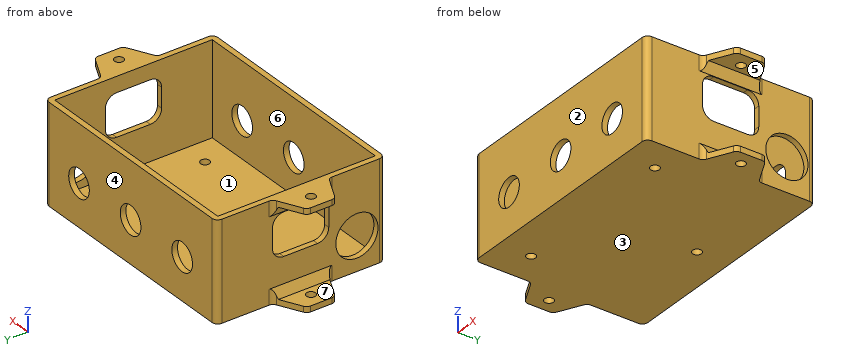
Autodesk Inventor part; units mm, degrees
ref_plane "Plano de trabajo1" through (41.5, -14.7294, 17.5) normal (0, 0, 1) x (1, 0, 0)
ref_plane "YZ Plane" through (0, 0, 0) normal (1, 0, 0) x (0, 1, 0)
ref_plane "XZ Plane" through (0, 0, 0) normal (0, 1, 0) x (-1, 0, 0)
sketch "Base" plane through (0, 0, 0) normal (0, 0, 1) x (1, 0, 0)
  line L0 (-41.5, -30) -> (41.5, -30)
  line L1 (41.5, -30) -> (41.5, -11.2361)
  line L2 (41.5, 30) -> (-41.5, 30)
  line L3 (-41.5, -30) -> (41.5, 30) construction
  line L4 (41.5, -30) -> (-41.5, 30) construction
  line L5 (-39.5, -28) -> (39.5, -28)
  line L6 (39.5, -28) -> (39.5, 28)
  line L7 (39.5, 28) -> (-39.5, 28)
  line L8 (-39.5, 28) -> (-39.5, -28)
  circle A0 centre (-30, -18.5) radius 1.35
  circle A1 centre (30, -18.5) radius 1.35
  circle A2 centre (0, 18.5) radius 1.35
  line L9 (51.5, 3.7639) -> (51.5, -3.7639)
  line L10 (41.5, 5) -> (51.5, -5) construction
  line L11 (51.5, 5) -> (41.5, -5) construction
  line L12 (42.6056, -9.4472) -> (50.3944, -5.5528)
  line L13 (50.3944, 5.5528) -> (42.6056, 9.4472)
  arc A3 (51.5, 3.7639) -> (50.3944, 5.5528) centre (49.5, 3.7639) ccw
  arc A4 (50.3944, -5.5528) -> (51.5, -3.7639) centre (49.5, -3.7639) ccw
  arc A5 (42.6056, -9.4472) -> (41.5, -11.2361) centre (43.5, -11.2361) ccw
  line L14 (41.5, 11.2361) -> (41.5, 30)
  arc A6 (41.5, 11.2361) -> (42.6056, 9.4472) centre (43.5, 11.2361) ccw
  line L15 (-41.5, -30) -> (-41.5, -11.2361)
  line L16 (-39.5, -28) -> (-39.5, 28)
  line L17 (-51.5, 3.7639) -> (-51.5, -3.7639)
  line L18 (-41.5, 5) -> (-51.5, -5) construction
  line L19 (-51.5, 5) -> (-41.5, -5) construction
  line L20 (-42.6056, -9.4472) -> (-50.3944, -5.5528)
  line L21 (-50.3944, 5.5528) -> (-42.6056, 9.4472)
  arc A7 (-50.3944, 5.5528) -> (-51.5, 3.7639) centre (-49.5, 3.7639) ccw
  arc A8 (-51.5, -3.7639) -> (-50.3944, -5.5528) centre (-49.5, -3.7639) ccw
  arc A9 (-41.5, -11.2361) -> (-42.6056, -9.4472) centre (-43.5, -11.2361) ccw
  line L22 (-41.5, 11.2361) -> (-41.5, 30)
  arc A10 (-42.6056, 9.4472) -> (-41.5, 11.2361) centre (-43.5, 11.2361) ccw
  line L23 (41.5, 11.2361) -> (41.5, -11.2361)
  line L24 (-41.5, -11.2361) -> (-41.5, 11.2361)
  circle A11 centre (-46.5, 0) radius 1.35
  circle A12 centre (46.5, 0) radius 1.35
  circle A13 centre (0, 18.5) radius 1.6
  circle A14 centre (30, -18.5) radius 1.6
  circle A15 centre (-30, -18.5) radius 1.6
  circle A16 centre (-46.5, 0) radius 1.6
  circle A17 centre (46.5, 0) radius 1.6
  point P0 (0, 0)
  point P1 (41.5, 10)
  point P2 (-41.5, 10)
  point P3 (-41.5, -10)
  point P4 (-41.5, 10)
  dimension "d0" = 83
  dimension "d1" = 60
  dimension "d5" = 2.7
  dimension "d6" = 9.5
  dimension "d8" = 2.7
  dimension "d9" = 5
  dimension "d10" = 10
  dimension "d11" = 10
  dimension "d14" = 2
  dimension "d15" = 2
  dimension "d16" = 2.7
  dimension "d17" = 2.7
  dimension "d63" = 3.2
  dimension "d64" = 3.2
  dimension "d65" = 3.2
  dimension "d66" = 3.2
  dimension "d67" = 3.2
extrude "Extrusión1" add sketch "Base" along normal blind 2 contours L8 L7 L6 L5 | A13 | A14 | A15
extrude "Extrusión2" add sketch "Base" along normal blind 2 contours A9 L20 A8 L17 A7 L21 A10 L24 | L23 A6 L13 A3 L9 A4 L12 A5 | A16 | A17
extrude "Extrusión3" cut sketch "Base" along normal blind 35 contours L15 L24 L22 L2 L14 L23 L1 L0
extrude "Extrusión4" add sketch "Base" along normal blind 35 contours L15 L24 L22 L2 L14 L23 L1 L0
sketch "Boceto2" plane through (-41.5, 30, 0) normal (0, 1, 0) x (1, 0, 0)
  line L0 (41.5, 0) -> (41.5, -35)
  line L1 (2, -35) -> (81, -35)
  line L2 (83, 0) -> (0, 0)
  circle A0 centre (16.5, -14.9) radius 5
  circle A1 centre (66.5, -14.9) radius 5
  circle A2 centre (41.5, -14.9) radius 5
  dimension "d26" = 14.9
  dimension "d27" = 25
  dimension "d28" = 10
  dimension "d29" = 10
extrude "Extrusión5" cut sketch "Boceto2" against normal blind 70
sketch "Boceto3" plane through (41.5, 11.2361, 0) normal (1, 0, 0) x (0, 0, -1)
  line L0 (-2, -39.2361) -> (-35, -39.2361)
  line L1 (-2, -15) -> (-2, -7.4721)
  line L2 (0, 0) -> (0, 18.7639)
  line L3 (-18.5, -21.2361) -> (-25.5, -21.2361)
  line L4 (-29.5, -17.2361) -> (-29.5, -5.2361)
  line L5 (-25.5, -1.2361) -> (-18.5, -1.2361)
  line L6 (-14.5, -5.2361) -> (-14.5, -17.2361)
  line L7 (-14.5, -21.2361) -> (-29.5, -1.2361) construction
  line L8 (-29.5, -21.2361) -> (-14.5, -1.2361) construction
  arc A0 (-29.5, -17.2361) -> (-25.5, -21.2361) centre (-25.5, -17.2361) ccw
  arc A1 (-18.5, -21.2361) -> (-14.5, -17.2361) centre (-18.5, -17.2361) ccw
  arc A2 (-14.5, -5.2361) -> (-18.5, -1.2361) centre (-18.5, -5.2361) ccw
  arc A3 (-25.5, -1.2361) -> (-29.5, -5.2361) centre (-25.5, -5.2361) ccw
  circle A4 centre (-12, 8.7639) radius 7.5
  point P0 (0, -11.2361)
  point P1 (-22, -11.2361)
  dimension "d32" = 28
  dimension "d33" = 48
  dimension "d34" = 20
  dimension "d35" = 12
  dimension "d36" = 15
  dimension "d37" = 20
  dimension "d38" = 4
  dimension "d39" = 15
extrude "Extrusión6" cut sketch "Boceto3" against normal blind 10
sketch3d "Boceto 3D1"
pattern_circular "Patrón circular1" count 2 over 360 about axis through (0, 0, 99.8627) along (0, 0, -1) of "Extrusión6"
sketch "Boceto4" plane through (41.5, 11.2361, 0) normal (1, 0, 0) x (0, 0, -1)
  line L0 (-35, -41.2361) -> (-35, 18.7639)
  point P0 (0, -11.2361)
  point P1 (-17.5, -25.9654)
  dimension "d45" = 17.5
ref_plane "Plano de trabajo1" through (41.5, -14.7294, 17.5) normal (0, 0, 1) x (1, 0, 0)
mirror "Simetría1" about plane through (41.5, -14.7294, 17.5) normal (0, 0, 1) of "Extrusión2"
chamfer "Chaflán1" distance 1.7 angle 63 1 edges at (41.5, 0, 33) measured on face at (43.0002, 0, 33)
mirror "Simetría2" about plane through (41.5, -14.7294, 17.5) normal (0, 0, 1) of "Extrusión2", "Simetría1", "Chaflán1"
chamfer "Chaflán2" distance 1.7 angle 63 1 edges at (-41.5, 0, 33) measured on face at (-43.0002, 0, 33)
chamfer "Chaflán3" distance 1.7 angle 63 1 edges at (-41.5, 0, 2) measured on face at (-43.0002, 0, 2)
fillet "Empalme1" radius 2 4 edges at (-41.5, 30, 17.5) (41.5, 30, 17.5) (41.5, -30, 17.5) (-41.5, -30, 17.5)
hole "Agujero2" at (0, 18.5, 0) at (-30, -18.5, 0) at (-46.5, 0, 0) at (30, -18.5, 0) at (46.5, 0, 0) direction (0, 0, 1) diameter 3.2 depth 23.25 tip angle 118
extrude "Extrusión8" cut sketch "Base" along normal blind 94.8 contours A16 | A17
properties part number "Contenedor del Arduino v1.1"
Input: part model. Units: mm. Frame: model coordinates. Face numbers are marked on the shaded views. A direction names the side the tool comes from. Give positions to 0.01 mm unless a question says otherwise; leave off trailing zeros. Loops run counter-clockwise (first coordinate to the right, second up) from the corner with the lowest first, then second, coordinate; pieces in that order, holes last. Notation, with made-up numbers: (51, 68) - (65, 68) arc R24 cw to (65, 104) - close; hole circle Ø6 at (26, -9). An arc over 180 degrees is marked (long way). Use CSV: the item, a comma, the result in double quotes. Start each with the question number.
Item 1: Mould query, pull axis Y, two halves, no side actions, for the marked faces 1, 2 and 3. Classes: pulls with the +Y half, pulls with the -Y half, needs draft (parallel to the pull), parting line crosses it, or undercut.
Item 2: Line query: line 1 (X direction, y = 0, z = 34); line 2 (X direction, y = 21.5, z = 20.5); line 3 (Y direction, x = 2.5, z = 4). Output: solid intervals per line, ascending.
Item 3: Reachability of the marked faces 4, 5, 6 and 7 from +Z, -Z, +X, -X, +Y, -Y: full face, straight path, thin tool, end or side. Return the list, or none.
Item 4: Section A-A on y = -14. Return loops of the section in (x, z), then the cut area to 3 significant figures.
Item 5: Section C-C on x = 13.5. Return loops of the section in (y, z), then the cut area to 3 significant figures.
Item 6: Section D-D on y = 7. Return loops of the section in (x, z), then the cut area to 3 significant figures.
Item 7: Contact query for flat-ended pins moving along their axis: P1, Ø6, axis at y = 18.5, z = 9, coming from the +X side; P2, Ø12, axis at y = -20, z = 12, coming from the +X side; P3, Ø3, axis at x = 46.5, y = 0, coming from the -Z side; P4, Ø0.6, axis at x = 40.5, z = 22.5, coming from the -Y side. Output: stop coordinate, or through.
Item 8: Section B-B on z = 23.5. Return loops of the section in (x, y).
Ans:
1,face 1,"undercut"
1,face 2,"pulls with the -Y half"
1,face 3,"needs draft"
2,line 1,"x = -51.5 to -48.1, -44.9 to -39.5, 39.5 to 44.9, 48.1 to 51.5"
2,line 2,"x = -41.5 to -39.5, 39.5 to 41.5"
2,line 3,"y = -30 to -28, 28 to 30"
3,face 4,"+Z, -Z, +X, -X, +Y"
3,face 5,"+X, +Y, -Y"
3,face 6,"+Z"
3,face 7,"-X, +Y, -Y"
4,outline,"(-41.5, 0) - (41.5, 0) - (41.5, 35) - (39.5, 35) - (39.5, 2) - (-39.5, 2) - (-39.5, 7.5) - (-41.5, 7.5) - close; (-41.5, 16.5) - (-39.5, 16.5) - (-39.5, 35) - (-41.5, 35) - close"
4,area,"280 mm2"
5,outline,"(-30, 0) - (30, 0) - (30, 35) - (28, 35) - (28, 2) - (-28, 2) - (-28, 35) - (-30, 35) - close"
5,area,"252 mm2"
6,outline,"(-47.5, 0) - (47.5, 0) - (47.5, 2) - (43.2, 2) - (41.5, 5.34) - (41.5, 14.63) - (39.5, 14.63) - (39.5, 2) - (-39.5, 2) - (-39.5, 14.63) - (-41.5, 14.63) - (-41.5, 5.34) - (-43.2, 2) - (-47.5, 2) - close; (-47.5, 33) - (-43.2, 33) - (-41.5, 29.66) - (-41.5, 29.37) - (-39.5, 29.37) - (-39.5, 35) - (-47.5, 35) - close; (39.5, 29.37) - (41.5, 29.37) - (41.5, 29.66) - (43.2, 33) - (47.5, 33) - (47.5, 35) - (39.5, 35) - close"
6,area,"298 mm2"
7,P1,"stops at x = -39.5"
7,P2,"stops at x = 41.5"
7,P3,"passes through"
7,P4,"stops at y = -29.87"
8,outline,"(-41.5, -28) arc R2 ccw to (-39.5, -30) - (39.5, -30) arc R2 ccw to (41.5, -28) - (41.5, -10) - (39.5, -10) - (39.5, -28) - (-39.5, -28) - (-39.5, -10) - (-41.5, -10) - close; (-41.5, 10) - (-39.5, 10) - (-39.5, 28) - (39.5, 28) - (39.5, 10) - (41.5, 10) - (41.5, 28) arc R2 ccw to (39.5, 30) - (-39.5, 30) arc R2 ccw to (-41.5, 28) - close"
